Can you work these out from the model? Positions are in its coordinate system, mm. A direction names the side the tool comes from. Coordinates: 2 decimals unless noted, no trailing zeros. Order: outer loops, then holes, each group sorted by start corner. A loop starts at its lowest first (then second) coordinate and runs counter-clockwise, first axis right, second up. Notation, with made-up numbers: (36.5, -19) - (49.5, -19) arc R7 ccw to (49.5, -14) - close; hole circle Ø11 at (1, 26.5). An arc over 180 degrees is marked (long way). Use a Markdown table: item, result. Add a question column.
(1) I want a section at C-C (z = -21). List the corners of the cut face in (x, y) for me, and give its area (3 significant figures).
(2) We'd pull the mould along X, two halves only. Please class faces 1 (the flat face through (-14.88, 21.73, -21.07)), 2 (the cylindrical face through (-2, 21, -1)), 3 (the cylindrical face through (-14.81, 15.18, -0.37)): pulls with the +X half, pulls with the -X half, needs draft (parallel to the pull), parting line crosses it, or undercut.
(3) If I drill on L1, parallel to X at y = 25, z = -53; L2, parallel to Z at x = -22.25, y = 16.75; L3, parallel to Z at x = -14.25, y = 21.25, over which ranges is the centre line in solid material (lowest first)? Write a range as [from, to].
(4) I want a section at D-D (y = 29). List the corners of the cut face in (x, z) for me, and give its area (3 significant figures).
(5) I want a section at A-A (y = 17.75). List the corners of the cut face in (x, z) for me.
(6) On a 3-axis mill with a long thin cutter (end or side, diameter ignored), from which of +Z, -Z, +X, -X, +Y, -Y can I reach the whole of each face in a straight line? I mean faces 4 (the cylindrical face through (-0.37, 15.18, -35.47)), 5 (the flat face through (-15.12, 21.73, -48.93)). Say none if no direction works.
Autodesk Inventor part; units mm, degrees
ref_plane "YZ Plane" through (0, 0, 0) normal (1, 0, 0) x (0, 1, 0)
ref_plane "XZ Plane" through (0, 0, 0) normal (0, 1, 0) x (-1, 0, 0)
ref_plane "XY Plane" through (0, 0, 0) normal (0, 0, 1) x (1, 0, 0)
sketch "Sketch1" plane through (0, 0, 0) normal (0, 1, 0) x (-1, 0, 0)
  line L0 (0, 0) -> (30, 0)
  line L1 (30, 0) -> (30, -70)
  line L2 (30, -70) -> (0, -70)
  line L3 (0, -70) -> (0, 0)
  dimension "d0" = 70
  dimension "d1" = 30
extrude "Extrusion1" add sketch "Sketch1" along normal blind 30
sketch "Sketch2" plane through (0, 30, 0) normal (0, 1, 0) x (1, 0, 0)
  line L0 (-30, 70) -> (-30, 0)
  line L1 (0, 70) -> (-30, 70)
  line L2 (-30, 0) -> (0, 0)
  line L3 (0, 0) -> (0, 70)
  line L4 (0, 70) -> (-30, 70)
  line L5 (-30, 70) -> (-30, 0)
  line L6 (-6.75, 6.75) -> (-23.25, 6.75)
  line L7 (-23.25, 6.75) -> (-23.25, 63.25)
  line L8 (-23.25, 63.25) -> (-6.75, 63.25)
  line L9 (-6.75, 63.25) -> (-6.75, 6.75)
  dimension "d4" = 16.5
extrude "Extrusion2" cut sketch "Sketch2" against normal blind 10 contours L6 L7 L8 L9
chamfer "Chamfer1" distance 10 angle 60 1 edges at (-15, 20, -63.25) measured on face at (-12.25, 23.3333, -63.25)
chamfer "Chamfer3" distance 10 angle 60 1 edges at (-15, 20, -6.75) measured on face at (-17.75, 23.3333, -6.75)
move faces "Move1" translate (0, -7.938, 0) faces at (-12.25, 20, -38.6432)
move faces "Move2" translate (0, 13, 0) faces at (-20, 0, -46.6667)
chamfer "Chamfer4" distance 2 angle 45 4 edges at (-15, 13, 0) (0, 13, -35) (-30, 13, -35) (-15, 13, -70)
fillet "Fillet1" radius 5 12 edges at (-30, 22.5, 0) (0, 22.5, 0) (0, 22.5, -70) (-30, 22.5, -70) (-15, 30, 0) (-30, 30, -35) (-15, 30, -70) (0, 30, -35) (-15, 15, 0) (0, 15, -35) (-15, 15, -70) (-30, 15, -35)
properties part number "CalibrationPlate"
Answers follow:
| question | item | result |
|---|---|---|
| 1 | outline | (-30, 17.07) arc R5 ccw to (-28.54, 13.54) - (-28, 13) - (-2, 13) - (-1.46, 13.54) arc R5 ccw to (0, 17.07) - (0, 25) arc R5 ccw to (-5, 30) - (-6.75, 30) - (-6.75, 21.77) - (-23.25, 21.77) - (-23.25, 30) - (-25, 30) arc R5 ccw to (-30, 25) - close |
| 1 | area | 358 mm² |
| 2 | face 1 | undercut |
| 2 | face 2 | pulls with the +X half |
| 2 | face 3 | needs draft |
| 3 | L1 | x = [-30, -23.25], [-6.75, 0] |
| 3 | L2 | z = [-69.99, -40.3], [-29.7, -0.01] |
| 3 | L3 | z = [-70, -48.09], [-21.91, 0] |
| 4 | outline | (-28, -65) arc R3 ccw to (-25, -68) - (-5, -68) arc R3 ccw to (-2, -65) - (-2, -5) arc R3 ccw to (-5, -2) - (-25, -2) arc R3 ccw to (-28, -5) - close; hole (-23.25, -61.52) - (-6.75, -61.52) - (-6.75, -8.48) - (-23.25, -8.48) - close |
| 4 | area | 833 mm² |
| 5 | outline | (-30, -65) arc R5 ccw to (-25, -70) - (-5, -70) arc R5 ccw to (0, -65) - (0, -5) arc R5 ccw to (-5, 0) - (-25, 0) arc R5 ccw to (-30, -5) - close; hole (-23.25, -42.03) - (-6.75, -42.03) - (-6.75, -27.97) - (-23.25, -27.97) - close |
| 6 | face 4 | +Z, -Z, +X, -Y |
| 6 | face 5 | +Y |
